```python
from build123d import *

# Parameters (mm, degrees)
F0_W     = 50
F0_H     = 32
F1_DEPTH = 32
F2_R     = 5
F3_R     = 11
F4_DEPTH = 5
F5_R     = 1
F6_DEPTH = 5


with BuildPart() as f1:
    # F0 (on Top) → F1 (new body)
    with BuildSketch(Plane.XY):
        Rectangle(F0_W, F0_H)
    extrude(amount=F1_DEPTH)

    # F2
    f2_edges = [f1.edges().sort_by_distance(p)[0] for p in [
        (-25, -16, 16),
        (-25, 16, 16),
        (25, -16, 16),
        (25, 16, 16),
    ]]
    fillet(f2_edges, radius=F2_R)

    # F3 (on face) → F4 (join)
    with BuildSketch(Plane.XY.offset(32)):
        with Locations((13.5, 0)):
            Circle(F3_R)
    extrude(amount=F4_DEPTH)

    # F5 (on face) → F6 (cut)
    with BuildSketch(Plane.XY.offset(37)):
        with Locations((21.5, 0)):
            Circle(F5_R)
        with Locations((13.5, 8)):
            Circle(F5_R)
        with Locations((5.5, 0)):
            Circle(F5_R)
        with Locations((13.5, -8)):
            Circle(F5_R)
    extrude(amount=-F6_DEPTH, mode=Mode.SUBTRACT)


solid = f1.part
```
Source: CAD feature listing. Evaluate the final solid. Frame: model axes, mm. A direction names the side the tool comes from. Round coordinates to 2 decimals unless told otherwise and drop trailing zeros. Loops run counter-clockwise (first coordinate to the right, second up) from the corner with the lowest first, then second, coordinate; pieces in that order, holes last. Notation, with made-up numbers: M 16,83.5 L 22,83.5 A17 ccw 22,90.5 Z; hole C 16,57.25 d6. An arc over 180 degrees is marked long. Use a Markdown table: item, result. Add a question column.
1. Line query: line 1 (Y direction, x = 13.5, z = 34.2); line 2 (Y direction, x = 13, z = 36); line 3 (Z direction, x = 1.5, y = 14). Output: solid intervals per line, ascending.
2. Contact query for a flat-ended pin moving along its axis: P1, Ø0.6, axis at x = 14, y = 8, coming from the +Z side. Output: stop coordinate, or through.
3. Section query C-C on x = 8. Return the cut outline in (y, z).
4. Mould query, pull axis Y, two halves, no side actions, for faces 3 (the cylindrical face through (-24, -14, 16)), 4 (the flat face through (0, 0, 0)), 5 (the flat face through (21, 0, 32)). Classes: pulls with the +Y half, pulls with the -Y half, needs draft (parallel to the pull), parting line crosses it, or undercut.
5. Section query A-A on y = 0. Return the cut outline in (x, z).
6. Section query B-B on x = 13.5. Return the cut outline in (y, z), then the cut area to 3 significant figures.
7. Reachability of faces 1 (the flat face through (5, 0, 32)), 2 (the cylindrical face through (23, -15, 16)) from +Z, -Z, +X, -X, +Y, -Y: full face, straight path, thin tool, end or side. Return the list, or none.
8. Section query D-D on y = -8. Return the cut outline in (x, z), then the cut area to 3 significant figures.
Reported:
| question | item | result |
|---|---|---|
| 1 | line 1 | y = -11 to -9, -7 to 7, 9 to 11 |
| 1 | line 2 | y = -10.99 to -8.87, -7.13 to 7.13, 8.87 to 10.99 |
| 1 | line 3 | z = 0 to 32 |
| 2 | P1 | stops at z = 32 |
| 3 | outline | M -16,0 L 16,0 L 16,32 L 9.53,32 L 9.53,37 L -9.53,37 L -9.53,32 L -16,32 Z |
| 4 | face 3 | pulls with the -Y half |
| 4 | face 4 | needs draft |
| 4 | face 5 | undercut |
| 5 | outline | M -25,0 L 25,0 L 25,32 L 24.5,32 L 24.5,37 L 22.5,37 L 22.5,32 L 20.5,32 L 20.5,37 L 6.5,37 L 6.5,32 L 4.5,32 L 4.5,37 L 2.5,37 L 2.5,32 L -25,32 Z |
| 6 | outline | M -16,0 L 16,0 L 16,32 L 11,32 L 11,37 L 9,37 L 9,32 L 7,32 L 7,37 L -7,37 L -7,32 L -9,32 L -9,37 L -11,37 L -11,32 L -16,32 Z |
| 6 | area | 1,110 mm² |
| 7 | face 1 | +Z |
| 7 | face 2 | +Z, -Z, +X, -Y |
| 8 | outline | M -25,0 L 25,0 L 25,32 L 21.05,32 L 21.05,37 L 14.5,37 L 14.5,32 L 12.5,32 L 12.5,37 L 5.95,37 L 5.95,32 L -25,32 Z |
| 8 | area | 1,670 mm² |
